Design review of the part built by this model. Coordinates are the model's own, in mm. Give positions to 0.01 mm unless a question says otherwise; leave off trailing zeros. Order: outer loops, then holes, each group sorted by start corner. A loop starts at its lowest first (then second) coordinate and runs counter-clockwise, first axis right, second up.
Autodesk Inventor part; units mm, degrees
ref_plane "YZ Plane" through (0, 0, 0) normal (1, 0, 0) x (0, 1, 0)
ref_plane "XZ Plane" through (0, 0, 0) normal (0, 1, 0) x (-1, 0, 0)
ref_plane "XY Plane" through (0, 0, 0) normal (0, 0, 1) x (1, 0, 0)
sketch "Sketch1" plane through (0, 0, 0) normal (0, 0, 1) x (1, 0, 0)
  circle A0 centre (0, 0) radius 7.62 construction
  circle A1 centre (0, 0) radius 9.75
  circle A2 centre (33.02, 0) radius 25.4 construction
  line L0 (0, 0) -> (7.62, 0)
  line L1 (0, 0) -> (7.62, 0) construction
  circle A3 centre (33.02, 0) radius 9.5
  line L2 (0, -30) -> (33.02, -30)
  line L3 (33.02, 30) -> (0, 30)
  arc A4 (33.02, -30) -> (63.02, 0) centre (33.02, 0) ccw
  arc A5 (0, 30) -> (0, -30) centre (0, 0) ccw
  circle A6 centre (0, 0) radius 25.4 construction
  line L4 (0, 25.4) -> (0, 0) construction
  line L5 (0, 25.4) -> (25.4, 25.4) construction
  circle A7 centre (0, 25.4) radius 2.2
  circle A8 centre (-21.997, 12.7) radius 2.2
  circle A9 centre (-21.997, -12.7) radius 2.2
  circle A10 centre (0, -25.4) radius 2.2
  circle A11 centre (21.997, -12.7) radius 2.2
  circle A12 centre (21.997, 12.7) radius 2.2
  line L6 (63.02, 0) -> (63.02, 30)
  line L7 (63.02, 30) -> (33.02, 30)
  circle A13 centre (58.02, 25) radius 2.2
  circle A14 centre (73.02, 0) radius 2.75
  circle A15 centre (73.02, 0) radius 10
  line L8 (81.02, 6) -> (63.02, 30)
  line L9 (78.02, -8.6603) -> (48.02, -25.9808)
  dimension "d13" = 50.8
  dimension "d0" = 15.24
  dimension "d1" = 19.5
  dimension "d2" = 50.8
  dimension "d3" = 7.62
  dimension "d4" = 0
  dimension "d5" = 33.02
  dimension "d6" = 19
  dimension "d9" = 30
  dimension "d10" = 60
  dimension "d14" = 25.4
  dimension "d15" = 90
  dimension "d16" = 4.4
  dimension "d19" = 360
  dimension "d21" = 30
  dimension "d22" = 30
  dimension "d26" = 90
  dimension "d28" = 4.4
  dimension "d29" = 5
  dimension "d30" = 5
  dimension "d38" = 5.5
  dimension "d39" = 10
  dimension "d40" = 20
extrude "Extrusion1" add sketch "Sketch1" along normal blind 7 contours A5 L3 L7 L6 A4 L2 | A4 A15 L9 | L6 L8 A15 | A15 | A11 | A12
fillet "Fillet2" radius 10 1 edges at (63.02, 30, 3.5)
properties part number "Inner Plate" material "Aluminum 6061"
1. For pin 1 (4 mm diameter, centred on x = 58.02, y = 25, fed in from -Z); pin 2 (4 mm diameter, centred on y = -15, z = 5, fed in from +X); pin 3 (3 mm diameter, centred on x = 70.5, z = 6, fed in from -Y); pin 4 (5.5 mm diameter, centred on x = 0, y = 25.4, fed in from +Z), all flat-tipped, find the tip position at first contact; note any pin that passes through.
Recorded:
pin 1: passes through
pin 2: stops at x = 70.5
pin 3: stops at y = -13.87
pin 4: stops at z = 7
2. Draft analysis for pull direction Y (two halves, no side actions). For faces 1 (the face through (56.274, 26.339, 3.451)), 2 (the face through (26, 7, 0)), 3 (the face through (23.53, -0.42, 3.45)), 4 (the face through (62.55, 28.915, 3.549)), state which applies: pulls with the +Y half, pulls with the -Y half, needs draft (parallel to the pull), parting line crosses it, or undercut.
Recorded:
face 1: undercut
face 2: needs draft
face 3: undercut
face 4: pulls with the +Y half
3. Take a section at D-D (z = 5.75). State how many separate pieces and enclosed holes the cut face has, then the cut area to 3 significant figures.
Recorded:
separate pieces: 1
enclosed holes: 8
area: 4,920 mm2
4. Take a section at B-B (x = 7). State the section outline as (y, z) points.
Recorded:
outline: (-30, 0) - (-6.79, 0) - (-6.79, 7) - (-30, 7) - close; (6.79, 0) - (30, 0) - (30, 7) - (6.79, 7) - close
5. Take a section at C-C (y = 12.7). State the section outline as (x, z) points (3 decimals).
Recorded:
outline: (-27.179, 0) - (-24.197, 0) - (-24.197, 7) - (-27.179, 7) - close; (-19.797, 0) - (75.995, 0) - (75.995, 7) - (-19.797, 7) - close
6. Take a section at A-A (y = 0). State the section outline as (x, z) points, then the cut area to 3 significant figures.
Recorded:
outline: (-30, 0) - (-9.75, 0) - (-9.75, 7) - (-30, 7) - close; (9.75, 0) - (23.52, 0) - (23.52, 7) - (9.75, 7) - close; (42.52, 0) - (70.27, 0) - (70.27, 7) - (42.52, 7) - close; (75.77, 0) - (83.02, 0) - (83.02, 7) - (75.77, 7) - close
area: 483 mm2
7. For line 1 along Y through (x, z) = (0, 2.5); line 2 along X through (y, z) = (1, 4.25); line 3 along X through (y, z) = (-7.5, 1.25), list the stretches that pass through material, from the lowest coordinate up.
Recorded:
line 1: y = -30 to -27.6, -23.2 to -9.75, 9.75 to 23.2, 27.6 to 30
line 2: x = -29.98 to -9.7, 9.7 to 23.57, 42.47 to 70.46, 75.58 to 82.97
line 3: x = -29.05 to -6.23, 6.23 to 27.19, 38.85 to 79.63
